Part model, mm, in its own coordinate system. A direction names the side the tool comes from. Give positions to 0.01 mm unless a question says otherwise; leave off trailing zeros. Order: outer loops, then holes, each group sorted by start corner. A loop starts at its lowest first (then second) coordinate and runs counter-clockwise, first axis right, second up. Notation, with made-up numbers: M 0,86.25 L 55,86.25 A13 ccw 55,101.25 Z; hole C 36.25,20 d3. An arc over 180 degrees is marked long. Answer as a JSON object with one key per item and string values.
from build123d import *

# Parameters (mm, degrees)
SKETCH022_W         = 115
SKETCH022_H         = 78
PAD010_DEPTH        = 8
HOLE002_D           = 3.4
HOLE002_DEPTH       = 8
HOLE002_CSINK_D     = 6.1
HOLE002_CSINK_ANGLE = 90
HOLE002_TIPS_R      = 1.7
SKETCH027_W         = 29
SKETCH027_H         = 29
POCKET009_DEPTH     = 1
SKETCH032_W         = 5
SKETCH032_H         = 48
SKETCH032_H_2       = 78
POCKET012_DEPTH     = 5


with BuildPart() as part:
    # Sketch022 (on Face1 of CopyPad011) → Pad010 (new body)
    with BuildSketch(Plane.XY.offset(24)):
        with Locations((52.5, 32)):
            Rectangle(SKETCH022_W, SKETCH022_H)
    extrude(amount=PAD010_DEPTH)

    # Hole002
    with Locations(Plane.XY.offset(32)):
        with Locations((-1, 67), (106, 67), (106, -3), (-1, -3), (32, 67), (73, -3), (32, -3), (73, 67)):
            CounterSinkHole(HOLE002_D / 2, HOLE002_CSINK_D / 2, depth=HOLE002_DEPTH, counter_sink_angle=HOLE002_CSINK_ANGLE)

    # Hole002 tips → Hole002 tip 1 section 0
    with BuildSketch(Plane.XY.offset(24), mode=Mode.PRIVATE) as hole002_tip_1_s0:
        with Locations((-1, 67)):
            Circle(HOLE002_TIPS_R)
    loft([hole002_tip_1_s0.sketch, Vertex(-1, 67, 22.978537)], mode=Mode.SUBTRACT)

    # Hole002 tips → Hole002 tip 2 section 0
    with BuildSketch(Plane.XY.offset(24), mode=Mode.PRIVATE) as hole002_tip_2_s0:
        with Locations((106, 67)):
            Circle(HOLE002_TIPS_R)
    loft([hole002_tip_2_s0.sketch, Vertex(106, 67, 22.978537)], mode=Mode.SUBTRACT)

    # Hole002 tips → Hole002 tip 3 section 0
    with BuildSketch(Plane.XY.offset(24), mode=Mode.PRIVATE) as hole002_tip_3_s0:
        with Locations((106, -3)):
            Circle(HOLE002_TIPS_R)
    loft([hole002_tip_3_s0.sketch, Vertex(106, -3, 22.978537)], mode=Mode.SUBTRACT)

    # Hole002 tips → Hole002 tip 4 section 0
    with BuildSketch(Plane.XY.offset(24), mode=Mode.PRIVATE) as hole002_tip_4_s0:
        with Locations((-1, -3)):
            Circle(HOLE002_TIPS_R)
    loft([hole002_tip_4_s0.sketch, Vertex(-1, -3, 22.978537)], mode=Mode.SUBTRACT)

    # Hole002 tips → Hole002 tip 5 section 0
    with BuildSketch(Plane.XY.offset(24), mode=Mode.PRIVATE) as hole002_tip_5_s0:
        with Locations((32, 67)):
            Circle(HOLE002_TIPS_R)
    loft([hole002_tip_5_s0.sketch, Vertex(32, 67, 22.978537)], mode=Mode.SUBTRACT)

    # Hole002 tips → Hole002 tip 6 section 0
    with BuildSketch(Plane.XY.offset(24), mode=Mode.PRIVATE) as hole002_tip_6_s0:
        with Locations((73, -3)):
            Circle(HOLE002_TIPS_R)
    loft([hole002_tip_6_s0.sketch, Vertex(73, -3, 22.978537)], mode=Mode.SUBTRACT)

    # Hole002 tips → Hole002 tip 7 section 0
    with BuildSketch(Plane.XY.offset(24), mode=Mode.PRIVATE) as hole002_tip_7_s0:
        with Locations((32, -3)):
            Circle(HOLE002_TIPS_R)
    loft([hole002_tip_7_s0.sketch, Vertex(32, -3, 22.978537)], mode=Mode.SUBTRACT)

    # Hole002 tips → Hole002 tip 8 section 0
    with BuildSketch(Plane.XY.offset(24), mode=Mode.PRIVATE) as hole002_tip_8_s0:
        with Locations((73, 67)):
            Circle(HOLE002_TIPS_R)
    loft([hole002_tip_8_s0.sketch, Vertex(73, 67, 22.978537)], mode=Mode.SUBTRACT)

    # Sketch027 → Pocket009 (cut)
    with BuildSketch(Plane(origin=(0, 0, 24), x_dir=(1, 0, 0), z_dir=(0, 0, -1))):
        with Locations((27.5, -16.5)):
            Rectangle(SKETCH027_W, SKETCH027_H)
    extrude(amount=-POCKET009_DEPTH, mode=Mode.SUBTRACT)

    # Sketch032 (on Face5 of Pocket009) → Pocket012 (cut)
    with BuildSketch(Plane.XY.offset(32)):
        with Locations((2.5, 32)):
            Rectangle(SKETCH032_W, SKETCH032_H)
        with Locations((12.5, 32)):
            Rectangle(SKETCH032_W, SKETCH032_H_2)
        with Locations((22.5, 32)):
            Rectangle(SKETCH032_W, SKETCH032_H_2)
        with Locations((32.5, 32)):
            Rectangle(SKETCH032_W, SKETCH032_H)
        with Locations((42.5, 32)):
            Rectangle(SKETCH032_W, SKETCH032_H_2)
        with Locations((52.5, 32)):
            Rectangle(SKETCH032_W, SKETCH032_H_2)
        with Locations((62.5, 32)):
            Rectangle(SKETCH032_W, SKETCH032_H_2)
        with Locations((72.5, 32)):
            Rectangle(SKETCH032_W, SKETCH032_H)
        with Locations((82.5, 32)):
            Rectangle(SKETCH032_W, SKETCH032_H_2)
        with Locations((92.5, 32)):
            Rectangle(SKETCH032_W, SKETCH032_H_2)
        with Locations((102.5, 32)):
            Rectangle(SKETCH032_W, SKETCH032_H)
    extrude(amount=-POCKET012_DEPTH, mode=Mode.SUBTRACT)


with BuildPart() as part_1:
    # Body002 placement: moved
    add(part.part.moved(Location((0, 0, -2.5))))


solid = part_1.part
1. Cut at A-A on x = 32. Give the cut face in (y, z), plus the area to 3 significant figures.
Worked answers:
{"outline": "M -7,21.5 L -4.7,21.5 L -4.7,28.15 L -6.05,29.5 L -7,29.5 Z; M -1.3,21.5 L 2,21.5 L 2,22.5 L 31,22.5 L 31,21.5 L 65.3,21.5 L 65.3,28.15 L 63.95,29.5 L 56,29.5 L 56,24.5 L 8,24.5 L 8,29.5 L 0.05,29.5 L -1.3,28.15 Z; M 68.7,21.5 L 71,21.5 L 71,29.5 L 70.05,29.5 L 68.7,28.15 Z", "area": "297 mm^2"}
2. Which spindle directions (+Z, -Z, +X, -X, +Y, -Y) get a long thin tool onto all of the face, cutting with end or side? Do faces 1 (the flat face through (2, 8, 27)), 2 (the flat face through (52, 33, 24.5)), 3 (the flat face through (47, 33, 29.5)). Say none if no direction does.
Worked answers:
{"face 1": "+Z", "face 2": "+Z, +Y, -Y", "face 3": "+Z, +X, -X, +Y, -Y"}
3. Cut at B-B on z = 26.25. State how many separate pieces and enclosed holes the cut face has, plus the area to 3 significant figures.
Worked answers:
{"separate pieces": "8", "enclosed holes": "12", "area": "5,210 mm^2"}
4. Pin check, flat tips, straight feed: P1, Ø4, axis at x = 72.5, y = 26, coming from the +Z side; P2, Ø5, axis at x = 14, y = 21.5, coming from the +Z side. Stop position of each tip, or through.
Worked answers:
{"P1": "stops at z = 24.5", "P2": "stops at z = 29.5"}
5. Cut at D-D on x = 73. Give the cut face in (y, z), plus the area to 3 significant figures.
Worked answers:
{"outline": "M -7,21.5 L -4.7,21.5 L -4.7,28.15 L -6.05,29.5 L -7,29.5 Z; M -1.3,21.5 L 65.3,21.5 L 65.3,28.15 L 63.95,29.5 L 56,29.5 L 56,24.5 L 8,24.5 L 8,29.5 L 0.05,29.5 L -1.3,28.15 Z; M 68.7,21.5 L 71,21.5 L 71,29.5 L 70.05,29.5 L 68.7,28.15 Z", "area": "326 mm^2"}
6. Two-plate mould, pull along X, no slides. Class faces 4 (the flat face through (95, 31, 27)), 5 (the flat face through (36, 33, 29.5)): +X half, -X half, draft (parallel to the pull), parting line (faces both ways), or undercut.
Worked answers:
{"face 4": "undercut", "face 5": "draft"}
7. Probe line 1 along Y through (x, z) = (-1, 26.75); line 2 along X through (y, z) = (67, 23.25); line 3 along Y through (x, z) = (73, 26.75). List the from-to ranges inside material, lowest first.
Worked answers:
{"line 1": "y = -7 to -4.7, -1.3 to 65.3, 68.7 to 71", "line 2": "x = -5 to -2.7, 0.7 to 30.3, 33.7 to 71.3, 74.7 to 104.3, 107.7 to 110", "line 3": "y = -7 to -4.7, -1.3 to 8, 56 to 65.3, 68.7 to 71"}
